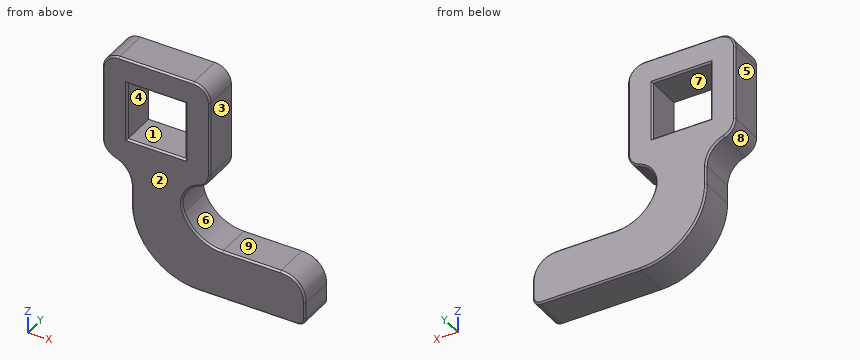
```python
from build123d import *

# Parameters (mm, degrees)
SKETCH_1_W      = 7
SKETCH_1_H      = 7
EXTRUDE_1_DEPTH = 4.5
SKETCH_4_W      = 6
SKETCH_4_H      = 4.5
EXTRUDE_4_DEPTH = 15
FILLET_1_SIZE   = 3
FILLET_3_R      = 5
FILLET_4_R      = 8
FILLET_5_R      = 2
FILLET_6_R      = 3
FILLET_7_R      = 1
CHAMFER_3_SIZE  = 0.2


with BuildPart() as part:
    # 草图1 → 凸台-拉伸1 (new body)
    with BuildSketch(Plane(origin=(0, 0, 0), x_dir=(1, 0, 0), z_dir=(0, 1, 0))):
        Polygon((9.5, 13), (13, 13), (13, 0), (0, 0), (0, 13), (3.5, 13), (3.5, 26), (9.5, 26), align=None)
        with Locations((6.5, 6.5)):
            Rectangle(SKETCH_1_W, SKETCH_1_H, mode=Mode.SUBTRACT)
    extrude(amount=EXTRUDE_1_DEPTH)

    # 草图4 → 凸台-拉伸4 (add)
    with BuildSketch(Plane(origin=(9.5, 0, 0), x_dir=(0, 0, -1), z_dir=(1, 0, 0))):
        with Locations((23, 2.25)):
            Rectangle(SKETCH_4_W, SKETCH_4_H)
    extrude(amount=EXTRUDE_4_DEPTH)

    # 圆角1
    # a fillet whose section is not a circle: 3 mm, written as the material it takes off along each edge
    with BuildSketch(Plane(origin=(24.5, 12, -20), x_dir=(-1, 0, 0), z_dir=(0, -1, 0))) as fillet_1_piece_1:
        with BuildLine():
            Bezier((FILLET_1_SIZE, 0), (0, 0), (0, FILLET_1_SIZE), weights=[1, 0.818181818, 1])
            Line((0, FILLET_1_SIZE), (0, 0))
            Line((0, 0), (FILLET_1_SIZE, 0))
        make_face()
    extrude(amount=19.5, mode=Mode.SUBTRACT)

    # 圆角3
    fillet_3_edges = [part.edges().sort_by_distance(p)[0] for p in [
        (9.5, 2.25, -20),
    ]]
    fillet(fillet_3_edges, radius=FILLET_3_R)

    # 圆角4
    fillet_4_edges = [part.edges().sort_by_distance(p)[0] for p in [
        (3.5, 2.25, -26),
    ]]
    fillet(fillet_4_edges, radius=FILLET_4_R)

    # 圆角5
    fillet_5_edges = [part.edges().sort_by_distance(p)[0] for p in [
        (0, 2.25, -13),
        (13, 2.25, -13),
        (13, 2.25, 0),
        (0, 2.25, 0),
    ]]
    fillet(fillet_5_edges, radius=FILLET_5_R)

    # 圆角6
    fillet_6_edges = [part.edges().sort_by_distance(p)[0] for p in [
        (9.5, 2.25, -13),
        (3.5, 2.25, -13),
    ]]
    fillet(fillet_6_edges, radius=FILLET_6_R)

    # 圆角7
    fillet_7_edges = [part.edges().sort_by_distance(p)[0] for p in [
        (24.5, 2.25, -26),
    ]]
    fillet(fillet_7_edges, radius=FILLET_7_R)

    # 倒角3
    chamfer_3_edges = [part.edges().sort_by_distance(p)[0] for p in [
        (18, 4.5, -20),
        (11.676872614, 4.5, -19.126736212),
        (11.676872614, 0, -19.126736212),
        (12.629227016, 0, -12.160008331),
        (12.629227016, 4.5, -12.160008331),
        (13, 4.5, -6.5),
        (13, 0, -6.5),
        (12.414213562, 4.5, -0.585786438),
        (12.414213562, 0, -0.585786438),
        (6.5, 0, 0),
        (6.5, 4.5, 0),
        (0.585786438, 4.5, -0.585786438),
        (0.585786438, 0, -0.585786438),
        (0, 0, -6.5),
        (0, 4.5, -6.5),
        (0.38754845, 4.5, -12.183215957),
        (0.38754845, 0, -12.183215957),
        (3.5, 0, -16.884848004),
        (3.5, 4.5, -16.884848004),
        (5.843145751, 4.5, -23.656854249),
        (5.843145751, 0, -23.656854249),
        (17.5, 4.5, -26),
        (17.5, 0, -26),
        (24.207106781, 0, -25.707106781),
        (24.207106781, 4.5, -25.707106781),
        (23.675, 4.5, -20.825),
        (23.675, 0, -20.825),
        (18, 0, -20),
        (10, 0, -6.5),
        (10, 4.5, -6.5),
        (6.5, 0, -3),
        (6.5, 4.5, -3),
        (3, 0, -6.5),
        (3, 4.5, -6.5),
        (6.5, 0, -10),
        (6.5, 4.5, -10),
        (2.918677324, 4.5, -13.994872072),
        (2.918677324, 0, -13.994872072),
        (9.913215245, 4.5, -14.465146968),
        (9.913215245, 0, -14.465146968),
        (24.5, 0, -24),
        (24.5, 4.5, -24),
    ]]
    chamfer(chamfer_3_edges, length=CHAMFER_3_SIZE)


solid = part.part
```
Model file for the job. Use its own axes, mm. Face numbers are marked on the shaded views. A direction names the side the tool comes from. Give positions to 0.01 mm unless a question says otherwise; leave off trailing zeros. Loops run counter-clockwise (first coordinate to the right, second up) from the corner with the lowest first, then second, coordinate; pieces in that order, holes last. Notation, with made-up numbers: (9, 74) - (40, 74) arc R17 cw to (40, 91) - close; hole circle Ø7 at (53, -38.75). An arc over 180 degrees is marked (long way). One line per item, written item: value. Start each with the question number.
1. Probe L1, parallel to X at y = 1.9, z = -4; L2, parallel to Z at x = 21.25, y = 3.35; L3, parallel to X at y = 4.35, z = -8.5. List the from-to ranges inside material, lowest first. Write a range as from..to.
2. Slice it at A-A (z = -8). List the corners of the cut face in (x, y), plus the area to 3 significant figures.
3. Pin check, flat tips, straight feed: pin 1 (2 mm diameter, centred on x = 5.5, z = -6.5, fed in from +Y); pin 2 (1.1 mm diameter, centred on y = 2.5, z = -16.5, fed in from -X); pin 3 (1.2 mm diameter, centred on y = 3, z = -7, fed in from +X); pin 4 (2 mm diameter, centred on x = 16.5, y = 3, fed in from +Z). Stop position of each tip, or through.
4. Which spindle directions (+Z, -Z, +X, -X, +Y, -Y) get a long thin tool onto all of the face, cutting with end or side? Do the marked faces 5, 6, 7, 8 and 9. Say none if no direction does.
5. Pull direction X, two halves, no side cores. Call the marked faces 1, 2, 3 and 4: pulls with the +X half, pulls with the -X half, needs draft (parallel to the pull), parting line crosses it, or undercut.
Solution:
1. L1: x = 0..3, 10..13
1. L2: z = -26..-20
1. L3: x = 0.05..2.95, 10.05..12.95
2. outline: (0, 0.2) - (0.2, 0) - (2.8, 0) - (3, 0.2) - (3, 4.3) - (2.8, 4.5) - (0.2, 4.5) - (0, 4.3) - close; (10, 0.2) - (10.2, 0) - (12.8, 0) - (13, 0.2) - (13, 4.3) - (12.8, 4.5) - (10.2, 4.5) - (10, 4.3) - close
2. area: 26.8 mm^2
3. pin 1: passes through
3. pin 2: stops at x = 3.5
3. pin 3: stops at x = 13
3. pin 4: stops at z = -20
4. face 5: +Z, -Z, -X, +Y, -Y
4. face 6: +X, +Y, -Y
4. face 7: +Y, -Y
4. face 8: -Z, -X, +Y, -Y
4. face 9: +Z, +X, +Y, -Y
5. face 1: undercut
5. face 2: needs draft
5. face 3: pulls with the +X half
5. face 4: undercut
